Could you check a few things on this model? Use its own coordinates, in mm. Round coordinates to 2 decimals unless told otherwise and drop trailing zeros. Order: outer loops, then holes, each group sorted by start corner. A loop starts at its lowest first (then second) coordinate and runs counter-clockwise, first axis right, second up. Notation, with made-up numbers: (76, 36) - (134, 36) arc R13 cw to (134, 49) - close; hole circle Ø9 at (6.5, 20). An arc over 180 degrees is marked (long way). Use one line per item in the form item = value.
from build123d import *

# Parameters (mm, degrees)
SKETCH1_W           = 120
SKETCH1_H           = 110
BOSS_EXTRUDE1_DEPTH = 3
SKETCH2_R           = 1.6
CUT_EXTRUDE1_DEPTH  = 4
SKETCH3_R           = 18
CUT_EXTRUDE2_DEPTH  = 10
CUT_EXTRUDE3_DEPTH  = 10
SKETCH5_R           = 1.6
CUT_EXTRUDE5_DEPTH  = 10
SKETCH6_R           = 3.5
SKETCH6_R_2         = 3.75
CUT_EXTRUDE6_DEPTH  = 10
SKETCH9_W           = 110
SKETCH9_H           = 3
BOSS_EXTRUDE2_DEPTH = 32
SKETCH8_R           = 1.6
CUT_EXTRUDE8_DEPTH  = 10


with BuildPart() as part:
    # Sketch1 → Boss-Extrude1 (new body)
    with BuildSketch(Plane(origin=(0, 0, 0), x_dir=(1, 0, 0), z_dir=(0, 1, 0))):
        Rectangle(SKETCH1_W, SKETCH1_H)
    extrude(amount=BOSS_EXTRUDE1_DEPTH)

    # Sketch2 → Cut-Extrude1 (cut)
    with BuildSketch(Plane(origin=(0, 3, 0), x_dir=(1, 0, 0), z_dir=(0, 1, 0))):
        with Locations(Location((19.25, 30, 0), (0, 0, 270))):
            Circle(SKETCH2_R)
        with Locations(Location((49.25, 30, 0), (0, 0, 270))):
            Circle(SKETCH2_R)
        with Locations(Location((-40, -14.25, 0), (0, 0, 270))):
            Circle(SKETCH2_R)
        with Locations(Location((-40, -44.25, 0), (0, 0, 270))):
            Circle(SKETCH2_R)
        with Locations(Location((0.75, 30, 0), (0, 0, 270))):
            Circle(SKETCH2_R)
        with Locations(Location((30.75, 30, 0), (0, 0, 270))):
            Circle(SKETCH2_R)
        with Locations(Location((-40, -25.75, 0), (0, 0, 270))):
            Circle(SKETCH2_R)
        with Locations(Location((-40, 4.25, 0), (0, 0, 270))):
            Circle(SKETCH2_R)
        with Locations(Location((-47.75, -5, 0), (0, 0, 270))):
            Circle(SKETCH2_R)
        with Locations(Location((-32.25, -5, 0), (0, 0, 270))):
            Circle(SKETCH2_R)
        with Locations(Location((-47.75, -35, 0), (0, 0, 270))):
            Circle(SKETCH2_R)
        with Locations(Location((-32.25, -35, 0), (0, 0, 270))):
            Circle(SKETCH2_R)
        with Locations(Location((10, 22.25, 0), (0, 0, 270))):
            Circle(SKETCH2_R)
        with Locations(Location((10, 37.75, 0), (0, 0, 270))):
            Circle(SKETCH2_R)
        with Locations(Location((40, 22.25, 0), (0, 0, 270))):
            Circle(SKETCH2_R)
        with Locations(Location((40, 37.75, 0), (0, 0, 270))):
            Circle(SKETCH2_R)
    extrude(amount=-CUT_EXTRUDE1_DEPTH, mode=Mode.SUBTRACT)

    # Sketch3 → Cut-Extrude2 (cut)
    with BuildSketch(Plane(origin=(0, 3, 0), x_dir=(1, 0, 0), z_dir=(0, 1, 0))):
        with Locations(Location((25, -20, 0), (0, 0, 270))):
            Circle(SKETCH3_R)
    extrude(amount=-CUT_EXTRUDE2_DEPTH, mode=Mode.SUBTRACT)

    # Sketch4 → Cut-Extrude3 (cut)
    with BuildSketch(Plane(origin=(0, 3, 0), x_dir=(1, 0, 0), z_dir=(0, 1, 0))):
        with BuildLine():
            Line((-41.6, -14.25), (-41.6, -10.25))
            ThreePointArc((-41.6, -10.25), (-40, -8.65), (-38.4, -10.25))
            Line((-38.4, -10.25), (-38.4, -14.25))
            ThreePointArc((-38.4, -14.25), (-40, -15.85), (-41.6, -14.25))
        make_face()
        with BuildLine():
            Line((-41.6, 4.25), (-41.6, 8.25))
            ThreePointArc((-41.6, 8.25), (-40, 9.85), (-38.4, 8.25))
            Line((-38.4, 8.25), (-38.4, 4.25))
            ThreePointArc((-38.4, 4.25), (-40, 2.65), (-41.6, 4.25))
        make_face()
        with BuildLine():
            Line((19.25, 28.4), (15.25, 28.4))
            ThreePointArc((15.25, 28.4), (13.65, 30), (15.25, 31.6))
            Line((15.25, 31.6), (19.25, 31.6))
            ThreePointArc((19.25, 31.6), (20.85, 30), (19.25, 28.4))
        make_face()
        with BuildLine():
            Line((0.75, 28.4), (-3.25, 28.4))
            ThreePointArc((-3.25, 28.4), (-4.85, 30), (-3.25, 31.6))
            Line((-3.25, 31.6), (0.75, 31.6))
            ThreePointArc((0.75, 31.6), (2.35, 30), (0.75, 28.4))
        make_face()
        with BuildLine():
            Line((-33.85, -5), (-33.85, -1))
            ThreePointArc((-33.85, -1), (-32.25, 0.6), (-30.65, -1))
            Line((-30.65, -1), (-30.65, -5))
            ThreePointArc((-30.65, -5), (-32.25, -6.6), (-33.85, -5))
        make_face()
        with BuildLine():
            Line((-49.35, -5), (-49.35, -1))
            ThreePointArc((-49.35, -1), (-47.75, 0.6), (-46.15, -1))
            Line((-46.15, -1), (-46.15, -5))
            ThreePointArc((-46.15, -5), (-47.75, -6.6), (-49.35, -5))
        make_face()
        with BuildLine():
            Line((10, 20.65), (6, 20.65))
            ThreePointArc((6, 20.65), (4.4, 22.25), (6, 23.85))
            Line((6, 23.85), (10, 23.85))
            ThreePointArc((10, 23.85), (11.6, 22.25), (10, 20.65))
        make_face()
        with BuildLine():
            Line((10, 36.15), (6, 36.15))
            ThreePointArc((6, 36.15), (4.4, 37.75), (6, 39.35))
            Line((6, 39.35), (10, 39.35))
            ThreePointArc((10, 39.35), (11.6, 37.75), (10, 36.15))
        make_face()
    extrude(amount=-CUT_EXTRUDE3_DEPTH, mode=Mode.SUBTRACT)

    # Sketch5 → Cut-Extrude5 (cut)
    with BuildSketch(Plane(origin=(0, 3, 0), x_dir=(1, 0, 0), z_dir=(0, 1, 0))):
        with Locations(Location((-56, 51, 0), (0, 0, 270))):
            Circle(SKETCH5_R)
        with Locations(Location((56, 51, 0), (0, 0, 270))):
            Circle(SKETCH5_R)
        with Locations(Location((56, -51, 0), (0, 0, 270))):
            Circle(SKETCH5_R)
        with Locations(Location((-56, -51, 0), (0, 0, 270))):
            Circle(SKETCH5_R)
    extrude(amount=-CUT_EXTRUDE5_DEPTH, mode=Mode.SUBTRACT)

    # Sketch6 → Cut-Extrude6 (cut)
    with BuildSketch(Plane(origin=(0, 3, 0), x_dir=(1, 0, 0), z_dir=(0, 1, 0))):
        with Locations(Location((-40, -35, 0), (0, 0, 270))):
            Circle(SKETCH6_R)
        with Locations(Location((40, 30, 0), (0, 0, 270))):
            Circle(SKETCH6_R_2)
        with BuildLine():
            Line((-43.5, -5), (-43.5, -1))
            ThreePointArc((-43.5, -1), (-40, 2.5), (-36.5, -1))
            Line((-36.5, -1), (-36.5, -5))
            ThreePointArc((-36.5, -5), (-40, -8.5), (-43.5, -5))
        make_face()
        with BuildLine():
            Line((10, 26.5), (6, 26.5))
            ThreePointArc((6, 26.5), (2.5, 30), (6, 33.5))
            Line((6, 33.5), (10, 33.5))
            ThreePointArc((10, 33.5), (13.5, 30), (10, 26.5))
        make_face()
    extrude(amount=-CUT_EXTRUDE6_DEPTH, mode=Mode.SUBTRACT)

    # Sketch9 → Boss-Extrude2 (add)
    with BuildSketch(Plane(origin=(60, 0, 0), x_dir=(0, 0, -1), z_dir=(1, 0, 0))):
        with Locations((0, 1.5)):
            Rectangle(SKETCH9_W, SKETCH9_H)
    extrude(amount=BOSS_EXTRUDE2_DEPTH)

    # Sketch8 → Cut-Extrude8 (cut)
    with BuildSketch(Plane.XZ):
        with Locations(Location((5.315, -6.608, 0), (0, 0, 270))):
            Circle(SKETCH8_R)
        with Locations(Location((5.315, 46.608, 0), (0, 0, 270))):
            Circle(SKETCH8_R)
        with Locations(Location((85.96, 46.608, 0), (0, 0, 270))):
            Circle(SKETCH8_R)
        with Locations(Location((85.96, -6.608, 0), (0, 0, 270))):
            Circle(SKETCH8_R)
    extrude(amount=-CUT_EXTRUDE8_DEPTH, mode=Mode.SUBTRACT)


solid = part.part
Item 1: Imagine slicing it at B-B on z = -51. Please give me the cut outline in (x, y).
Found:
outline = (-60, 0) - (-57.6, 0) - (-57.6, 3) - (-60, 3) - close; (-54.4, 0) - (54.4, 0) - (54.4, 3) - (-54.4, 3) - close; (57.6, 0) - (92, 0) - (92, 3) - (57.6, 3) - close
Item 2: If we mould it in two halves opening along X, with no side actions, what happens to faces 1 (the face through (-41.42, 1.52, 26.49)), 2 (the face through (5.385, 1.479, 48.206))? For each: released by +X, released by -X, zero draft, split by the parting line, or undercut.
Found:
face_1 = undercut
face_2 = undercut
Item 3: Imagine slicing it at A-A on x = 85.96. Please give me the cut outline in (y, z).
Found:
outline = (0, -55) - (3, -55) - (3, -8.21) - (0, -8.21) - close; (0, -5.01) - (3, -5.01) - (3, 45.01) - (0, 45.01) - close; (0, 48.21) - (3, 48.21) - (3, 55) - (0, 55) - close
Item 4: I need wall thicknesses on L1, parallel to X at y = 1.5, z = -37.75; L2, parallel to X at y = 2.2, z = 51; L3, parallel to Z at x = -43, y = 0.45. Which ranges of each line are inside material? Lowest first, please.
Found:
L1 = -60 to 4.4, 11.6 to 38.4, 41.6 to 92
L2 = -60 to -57.6, -54.4 to 54.4, 57.6 to 92
L3 = -55 to -0.8, 6.8 to 33.2, 36.8 to 55
Item 5: Imagine slicing it at C-C on z = 35. Please give me the cut outline in (x, y).
Found:
outline = (-60, 0) - (-49.35, 0) - (-49.35, 3) - (-60, 3) - close; (-46.15, 0) - (-43.5, 0) - (-43.5, 3) - (-46.15, 3) - close; (-36.5, 0) - (-33.85, 0) - (-33.85, 3) - (-36.5, 3) - close; (-30.65, 0) - (15.05, 0) - (15.05, 3) - (-30.65, 3) - close; (34.95, 0) - (92, 0) - (92, 3) - (34.95, 3) - close
Item 6: Imagine slicing it at D-D on y = 2.5. State how many separate pieces and enclosed holes the cut face has, plus the area to 3 significant figures.
Found:
separate_pieces = 1
enclosed_holes = 29
area = 15,200 mm2
